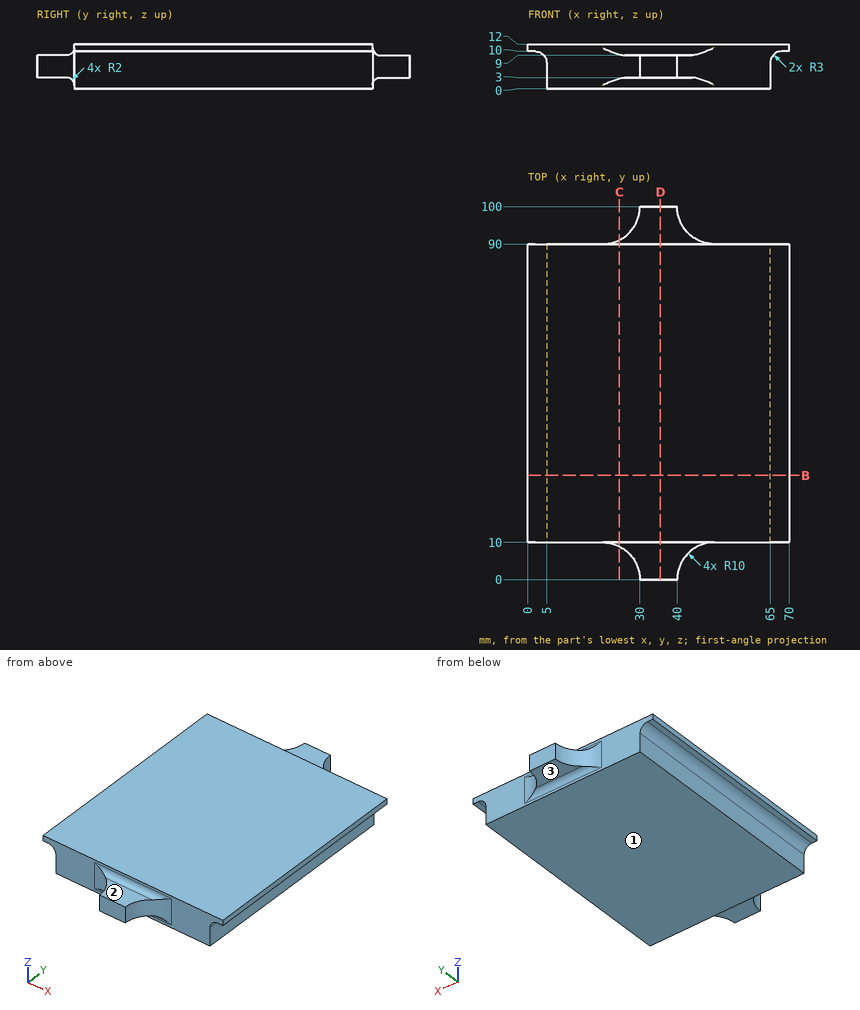
Geometry: see drawing. Coordinates: mm, zero at the bounding-box minimum. A direction names the side the tool comes from. Round coordinates to 2 decimals unless told otherwise and drop trailing zeros. Loops run counter-clockwise (first coordinate to the right, second up) from the corner with the lowest first, then second, coordinate; pieces in that order, holes last. Notation, with made-up numbers: M 7,-38 L 19,-38 A16 cw 19,-20 Z; hole C 34.5,-30 d3. An arc over 180 degrees is marked long. Use a Markdown table: item, result. Add a question column.
1. Contact query for flat-ended pins moving along their axis: pin 1 (4 mm diameter, centred on x = 38, y = 97.5, fed in from +Z); pin 2 (2 mm diameter, centred on x = 0.5, y = 30.5, fed in from -Z); pin 3 (6 mm diameter, centred on x = 21.5, z = 3, fed in from +Y). Output: stop coordinate, or through.
2. Ray query, line 1 along X through (y, z) = (25.5, 3.75); line 2 along X through (y, z) = (8, 8.75); line 3 along Y through (x, z) = (6.5, 7.5). Return the intervals inside material, ascending. Write a range as [from, to].
3. Cut plane C-C, the plane x = 24.5. Output: boundary loops of the cut face in (y, z), and give its area (3 significant figures).
4. Cut plane B-B, the plane y = 28. Output: boundary loops of the cut face in (x, z), and give its area (3 significant figures).
5. Set-up query: the marked faces 1, 2 and 3. Return all of +Z, -Z, +X, -X, +Y, -Y with unobstructed straight access to the full face (end or side cutting, diameter ignored); none if empty.
6. Cut plane D-D, the plane x = 35.5. Output: boundary loops of the cut face in (y, z).
Solution:
| question | item | result |
|---|---|---|
| 1 | pin 1 | stops at z = 9 |
| 1 | pin 2 | stops at z = 10 |
| 1 | pin 3 | stops at y = 91.07 |
| 2 | line 1 | x = [5, 65] |
| 2 | line 2 | x = [26, 44] |
| 2 | line 3 | y = [10, 90] |
| 3 | outline | M 8.93,2.77 A2 cw 10,1 L 10,0 L 90,0 L 90,1 A2 cw 91.07,2.77 L 91.07,9.23 A2 cw 90,11 L 90,12 L 10,12 L 10,11 A2 cw 8.93,9.23 Z |
| 3 | area | 976 mm2 |
| 4 | outline | M 0,10 L 2,10 A3 cw 5,7 L 5,0 L 65,0 L 65,7 A3 cw 68,10 L 70,10 L 70,12 L 0,12 Z |
| 4 | area | 744 mm2 |
| 5 | face 1 | -Z, +X, -X, +Y, -Y |
| 5 | face 2 | +Z, +X, -X, -Y |
| 5 | face 3 | -Z, +X, -X, +Y |
| 6 | outline | M 0,3 L 8,3 A2 cw 10,1 L 10,0 L 90,0 L 90,1 A2 cw 92,3 L 100,3 L 100,9 L 92,9 A2 cw 90,11 L 90,12 L 10,12 L 10,11 A2 cw 8,9 L 0,9 Z |
